from build123d import *

# Parameters (mm, degrees)
F1_DEPTH = 12.7
F2_R     = 3.175
F3_DEPTH = 25.4
F4_DEPTH = 6.35
F6_DEPTH = 25.4


with BuildPart() as f1:
    # F0 (on Top) → F1 (new body)
    with BuildSketch(Plane.XY):
        with BuildLine():
            Line((35.9911476828, 94.3723806679), (33.4511476828, 94.3723806679))
            Line((33.4511476828, 94.3723806679), (33.4511476828, -70.7276193321))
            Line((33.4511476828, -70.7276193321), (46.1511476828, -70.7276193321))
            Line((46.1511476828, -70.7276193321), (46.1511476828, -30.0876193321))
            ThreePointArc((46.1511476828, -30.0876193321), (38.9669427859, -27.1118242289), (35.9911476828, -19.9276193321))
            Line((35.9911476828, -19.9276193321), (35.9911476828, 94.3723806679))
        make_face()
    extrude(amount=F1_DEPTH)

    # F2 (on face) → F3 (cut)
    with BuildSketch(Plane(origin=(33.4511476828, 0, 0), x_dir=(0, -1, 0), z_dir=(-1, 0, 0))):
        with Locations((58.0276193321, 6.35)):
            Circle(F2_R)
        with Locations((38.9776193321, 6.35)):
            Circle(F2_R)
    extrude(amount=-F3_DEPTH, mode=Mode.SUBTRACT)

    # F4 (add): a face of the model
    f4_faces = [f1.faces().sort_by_distance(p)[0] for p in [
        (34.3352702719, 37.2223806679, 0),
    ]]
    extrude(f4_faces, amount=F4_DEPTH)

    # F5 (on face) → F6 (cut)
    with BuildSketch(Plane(origin=(33.4511476828, 0, 0), x_dir=(0, -1, 0), z_dir=(-1, 0, 0))):
        with BuildLine():
            Line((32.8058376908, 0), (-94.3723806679, 0))
            Line((-94.3723806679, 0), (-94.3723806679, -6.35))
            Line((-94.3723806679, -6.35), (39.1558376908, -6.35))
            ThreePointArc((39.1558376908, -6.35), (37.2959657514, -1.8598719395), (32.8058376908, 0))
        make_face()
    extrude(amount=-F6_DEPTH, mode=Mode.SUBTRACT)


solid = f1.part
The listing builds one solid part. Answer for the finished solid, in the listing's coordinates (mm). A direction names the side the tool comes from. Round coordinates to 2 decimals unless told otherwise and drop trailing zeros. Order: outer loops, then holes, each group sorted by start corner. A loop starts at its lowest first (then second) coordinate and runs counter-clockwise, first axis right, second up. Notation, with made-up numbers: M -32.5,-31.75 L 15.5,-31.75 A17 ccw 15.5,-0.75 Z; hole C 42.5,10.5 d10. An arc over 180 degrees is marked long. Answer in a Markdown table with one row per item. Add a question column.
1) Determine the mould class of faces 1 (the face through (39.712, -54.856, 6.49)), 2 (the face through (35, -24, 12.7)), 3 (the face through (35, 94.372, 6)), 4 (the face through (39.71, -36.64, 8.5)) for opening direction Y: pulls with the +Y half, pulls with the -Y half, needs draft (parallel to the pull), parting line crosses it, or undercut.
2) The part is cut by section B-B on x = 38.25. Determine the outline of the cut face in (y, z) (3 decimals).
3) The part is cut by section D-D on y = 77. Determine the outline of the cut face in (x, z).
4) Consider line 1 along X through (y, z) = (36, 1); line 2 along Y through (x, z) = (37.5, 5.5); line 3 along Z through (x, y) = (35.5, 71). Determine where each line is inside the solid, lowest interval first. Write a range as from..to.
5) The part is cut by section C-C on y = -37.5. Determine the outline of the cut face in (x, z), plus the area to 3 significant figures.
6) The part is cut by section A-A on z = 6.35. Determine the outline of the cut face in (x, y).
7) Which of the six approach directions +Z, -Z, +X, -X, +Y, -Y give full straight-line access (tool end or side, diameter ignored) to faces 5 (the face through (33.451, 13, 5)), 6 (the face through (35.991, 36, 6)), 7 (the face through (35.5, 21.1, 0))?
8) Flat-ended cylindrical pins translate along their axes: pin 1 Ø4 at (x, y) = (39.5, -30) entering from -Z; pin 2 Ø1.5 at (y, z) = (43.5, 6) entering from +X. Find the tip coordinate at first contact, or state that the pin passes through.
Findings below:
| question | item | result |
|---|---|---|
| 1 | face 1 | undercut |
| 1 | face 2 | needs draft |
| 1 | face 3 | pulls with the +Y half |
| 1 | face 4 | undercut |
| 2 | outline | M -70.728,-6.35 L -39.156,-6.35 A6.35 cw -32.806,0 L -26.315,0 L -26.315,12.7 L -70.728,12.7 Z; hole C -58.028,6.35 d6.35; hole C -38.978,6.35 d6.35 |
| 3 | outline | M 33.45,0 L 35.99,0 L 35.99,12.7 L 33.45,12.7 Z |
| 4 | line 1 | x = 33.45..35.99 |
| 4 | line 2 | y = -70.73..-61.09, -54.97..-42.04, -35.92..-25.26 |
| 4 | line 3 | z = 0..12.7 |
| 5 | outline | M 33.45,-2.07 L 46.15,-2.07 L 46.15,3.54 L 33.45,3.54 Z; M 33.45,9.16 L 46.15,9.16 L 46.15,12.7 L 33.45,12.7 Z |
| 5 | area | 116 mm² |
| 6 | outline | M 33.45,-70.73 L 46.15,-70.73 L 46.15,-61.2 L 33.45,-61.2 Z; M 33.45,-54.85 L 46.15,-54.85 L 46.15,-42.15 L 33.45,-42.15 Z; M 33.45,-35.8 L 46.15,-35.8 L 46.15,-30.09 A10.16 cw 35.99,-19.93 L 35.99,94.37 L 33.45,94.37 Z |
| 7 | face 5 | +Z, -Z, -X, +Y, -Y |
| 7 | face 6 | +Z, -Z, +X, +Y |
| 7 | face 7 | -Z, +X, -X, +Y |
| 8 | pin 1 | stops at z = 0 |
| 8 | pin 2 | stops at x = 35.99 |
